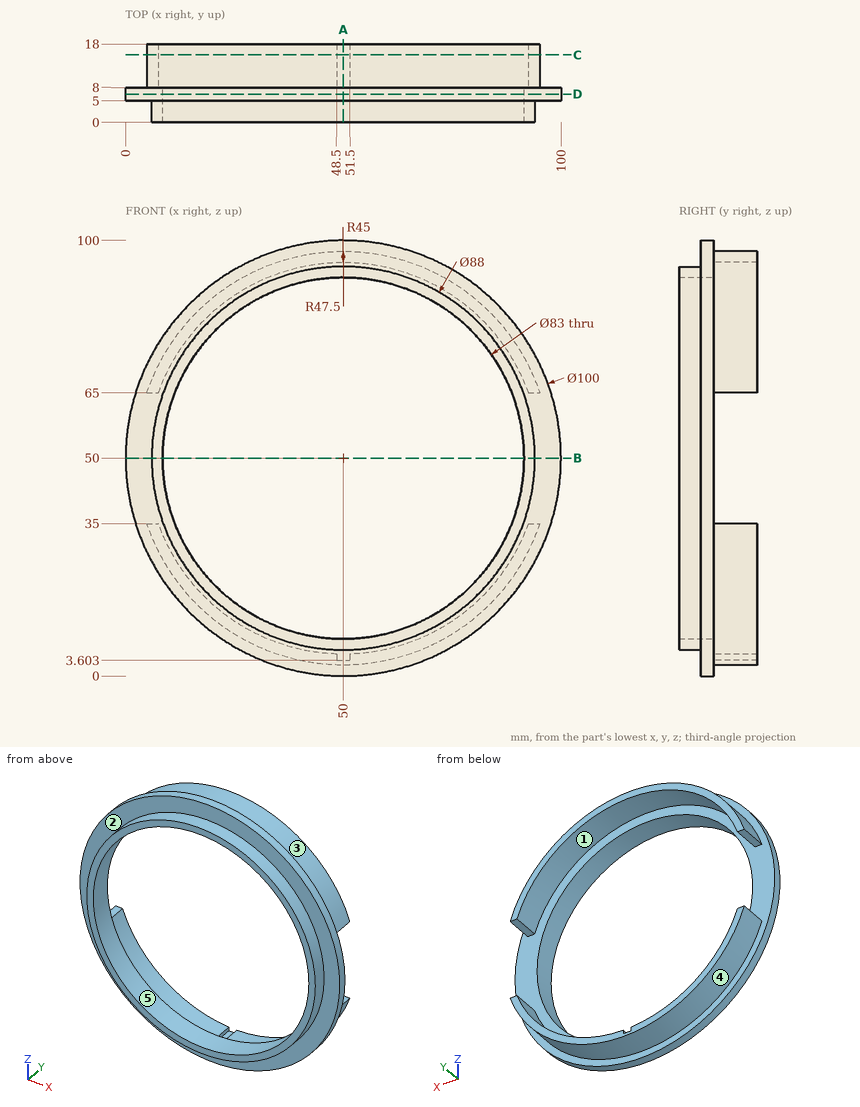
Job drawing, mm, ordinate dimensions from the low corner. One solid piece. A direction names the side the tool comes from. Round coordinates to 2 decimals unless told otherwise and drop trailing zeros. Loops run counter-clockwise (first coordinate to the right, second up) from the corner with the lowest first, then second, coordinate; pieces in that order, holes last.
(1) Wall check: line 1 along Z through (x, y) = (51, 1); line 2 along Z through (x, y) = (51, 17); line 3 along Y through (x, z) = (94, 72.5). Give the ranges that are in metal, low to high.
(2) Two-plate mould, pull along Z, no slides. Class the marked faces 1, 2 and 3: +Z half, -Z half, draft (parallel to the pull), parting line (faces both ways), or undercut.
(3) Cut at D-D (y = 6.5). Give the cut face in (x, z).
(4) Drop flat-ended pins along their axis: pin 1 (1.3 mm diameter, centred on x = 94, y = 14, fed in from -Z); pin 2 (2 mm diameter, centred on x = 89, y = 3, fed in from -Z); pin 3 (2 mm diameter, centred on x = 61, y = 6.5, fed in from -Z). Give the stop position or say it passes through.
(5) Which spindle directions (+Z, -Z, +X, -X, +Y, -Y) get a long thin tool onto all of the face, cutting with end or side? Do the marked faces 4 and 5. Say none if no direction does.
(6) Cut at B-B (z = 50). Give the cut face in (x, y), plus the area to 3 significant figures.
(7) Cut at C-C (y = 15.5). Give the cut face in (x, z) (1 decimal).
(8) Cut at A-A (x = 50). Give the cut face in (y, z).
Findings below:
1. line 1: z = 6.01 to 8.51, 91.49 to 93.99
1. line 2: z = 2.51 to 3.6, 94.99 to 97.49
1. line 3: y = 5 to 8
2. face 1: undercut
2. face 2: draft
2. face 3: +Z half
3. outline: circle Ø100 at (50, 50); hole circle Ø83 at (50, 50)
4. pin 1: stops at z = 30.58
4. pin 2: stops at z = 27.82
4. pin 3: stops at z = 1.01
5. face 4: -Z, +Y
5. face 5: +Y, -Y
6. outline: (0, 5) - (6, 5) - (6, 0) - (8.5, 0) - (8.5, 8) - (0, 8) - close; (91.5, 0) - (94, 0) - (94, 5) - (100, 5) - (100, 8) - (91.5, 8) - close
6. area: 76.0 mm2
7. outline: (4.9, 35) arc R47.5 ccw to (95.1, 35) - (92.4, 35) arc R45 cw to (51.5, 5) - (51.5, 3.6) - (48.5, 3.6) - (48.5, 5) arc R45 cw to (7.6, 35) - close; (4.9, 65) - (7.6, 65) arc R45 cw to (92.4, 65) - (95.1, 65) arc R47.5 ccw to start
8. outline: (0, 6) - (5, 6) - (5, 0) - (8, 0) - (8, 2.5) - (18, 2.5) - (18, 3.6) - (8, 3.6) - (8, 8.5) - (0, 8.5) - close; (0, 91.5) - (8, 91.5) - (8, 95) - (18, 95) - (18, 97.5) - (8, 97.5) - (8, 100) - (5, 100) - (5, 94) - (0, 94) - close
